Read the model definition and answer for the solid it produces. Units are mm, in the model's axes. Coordinates: 2 decimals unless noted, no trailing zeros. Write each loop counter-clockwise with the first axis right and the second up, starting at its lowest first coordinate (ties: lowest second). Pieces come first, ordered by that corner, then holes. Notation, with made-up numbers: (-9, -9) -> (47, -9) arc R14 ccw to (47, 17) -> close; hole circle Ø8 at (64, -14.5). An arc over 180 degrees is marked (long way). Answer as a JSON object with one key per item and string values. Group by question number.
(1) Find section A-A (x = 32). Give the vertices of the cut face in (y, z) (3 decimals), then the cut area to 3 significant figures.
(2) Find section D-D (x = 15). Give the vertices of the cut face in (y, z) (3 decimals).
(3) Straight lines are drawn through the part: L1, parallel to X at y = -12.3, z = 7.95; L2, parallel to X at y = -21, z = 5.25; L3, parallel to X at y = -7, z = 6.75. For each, find the intervals that lie inside material, in ascending order.
(4) Find section B-B (z = 2). Count the separate pieces of the cut face and the enclosed holes in it, then the cut area to 3 significant figures.
(5) A flat-ended cylindrical pin translates along its axis: P1, Ø7, axis at x = 15, y = -12.3, coming from the -Z side. Find the tip coordinate at first contact, or state that the pin passes through.
(6) Find section C-C (y = 4.68). Give the vertices of the cut face in (x, z) (1 decimal), then the cut area to 3 significant figures.
from build123d import *

# Parameters (mm, degrees)
F0_W           = 80
F0_H           = 50
F1_DEPTH       = 9.525
F4_DEPTH       = 25
F5_R           = 4.7625
F6_DEPTH       = 9.526
F7_D           = 5.5
F7_CBORE_D     = 9.75
F7_CBORE_DEPTH = 5


with BuildPart() as f1:
    # F0 (on Top) → F1 (new body)
    with BuildSketch(Plane.XY):
        Rectangle(F0_W, F0_H)
    extrude(amount=F1_DEPTH)

    # F3 (on face) → F4 (cut)
    with BuildSketch(Plane.XY.offset(9.525)):
        with BuildLine():
            ThreePointArc((-29.3, 18.9330952615), (-32, 21.6330952615), (-34.7, 18.9330952615))
            Line((-34.7, 18.9330952615), (-34.7, 8.9330952615))
            ThreePointArc((-34.7, 8.9330952615), (-32, 6.2330952615), (-29.3, 8.9330952615))
            Line((-29.3, 8.9330952615), (-29.3, 18.9330952615))
        make_face()
        with BuildLine():
            ThreePointArc((-34.7, -18.9330952615), (-32, -21.6330952615), (-29.3, -18.9330952615))
            Line((-29.3, -18.9330952615), (-29.3, -8.9330952615))
            ThreePointArc((-29.3, -8.9330952615), (-32, -6.2330952615), (-34.7, -8.9330952615))
            Line((-34.7, -8.9330952615), (-34.7, -18.9330952615))
        make_face()
        with BuildLine():
            ThreePointArc((29.3, -18.9330952615), (32, -21.6330952615), (34.7, -18.9330952615))
            Line((34.7, -18.9330952615), (34.7, -8.9330952615))
            ThreePointArc((34.7, -8.9330952615), (32, -6.2330952615), (29.3, -8.9330952615))
            Line((29.3, -8.9330952615), (29.3, -18.9330952615))
        make_face()
        with BuildLine():
            ThreePointArc((34.7, 18.9330952615), (32, 21.6330952615), (29.3, 18.9330952615))
            Line((29.3, 18.9330952615), (29.3, 8.9330952615))
            ThreePointArc((29.3, 8.9330952615), (32, 6.2330952615), (34.7, 8.9330952615))
            Line((34.7, 8.9330952615), (34.7, 18.9330952615))
        make_face()
    extrude(amount=-F4_DEPTH, mode=Mode.SUBTRACT)

    # F5 (on face) → F6 (cut, through all)
    with BuildSketch(Plane.XY.offset(9.525)):
        with Locations((0, 4.68)):
            Circle(F5_R)
    extrude(amount=-F6_DEPTH, mode=Mode.SUBTRACT)

    # F7 (through all)
    with Locations(Plane(origin=(0, 0, 0), x_dir=(1, 0, 0), z_dir=(0, 0, -1))):
        with Locations((-15, 12.3), (15, 12.3)):
            CounterBoreHole(F7_D / 2, F7_CBORE_D / 2, F7_CBORE_DEPTH)


solid = f1.part
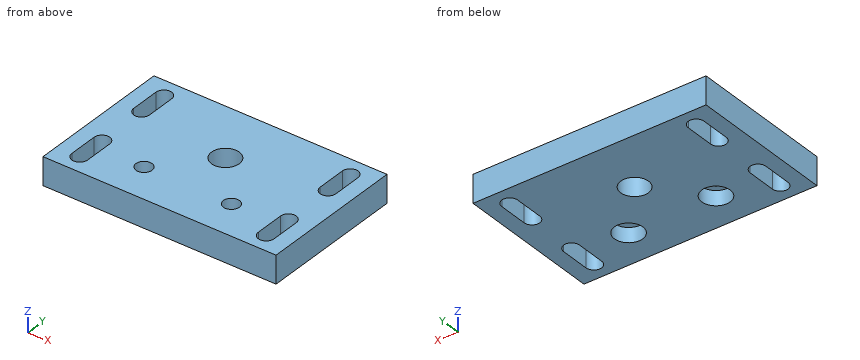
Results below:
{
 "1": {"outline": "(-25, 0) -> (-21.633, 0) -> (-21.633, 9.525) -> (-25, 9.525) -> close; (-6.233, 0) -> (6.233, 0) -> (6.233, 9.525) -> (-6.233, 9.525) -> close; (21.633, 0) -> (25, 0) -> (25, 9.525) -> (21.633, 9.525) -> close", "area": "183 mm2"},
 "2": {"outline": "(-25, 0) -> (-17.175, 0) -> (-17.175, 5) -> (-15.05, 5) -> (-15.05, 9.525) -> (-25, 9.525) -> close; (-9.55, 5) -> (-7.425, 5) -> (-7.425, 0) -> (25, 0) -> (25, 9.525) -> (-9.55, 9.525) -> close"},
 "3": {"L1": "x = -40 to -34.7, -29.3 to -17.75, -12.25 to 12.25, 17.75 to 29.3, 34.7 to 40", "L2": "x = -40 to -33.74, -30.26 to 30.26, 33.74 to 40", "L3": "x = -40 to -33.88, -30.12 to 30.12, 33.88 to 40"},
 "4": {"separate pieces": "1", "enclosed holes": "7", "area": "3,470 mm2"},
 "5": {"P1": "stops at z = 5"},
 "6": {"outline": "(-40, 0) -> (-4.8, 0) -> (-4.8, 9.5) -> (-40, 9.5) -> close; (4.8, 0) -> (40, 0) -> (40, 9.5) -> (4.8, 9.5) -> close", "area": "671 mm2"}
}
